```python
from build123d import *

# Parameters (mm, degrees)
F0_W     = 400
F0_H     = 80
F1_DEPTH = 7.5
F2_R     = 8
F3_W     = 12
F3_H     = 15
F3_W_2   = 15
F3_H_2   = 12
F4_DEPTH = 11.5
F5_R     = 5.5
F6_DEPTH = 25


# Not quite as in the source:
# - a pattern or mirror of a feature is missing from the dataset's text; its kind, count and spacing are read off the source's solid


with BuildPart() as f1:
    # F0 (on Top) → F1 (new body, symmetric)
    with BuildSketch(Plane.XY):
        Rectangle(F0_W, F0_H)
    extrude(amount=F1_DEPTH, both=True)

    # F2
    f2_edges = [f1.edges().sort_by_distance(p)[0] for p in [
        (-200, -40, 0),
        (200, -40, 0),
        (200, 40, 0),
        (-200, 40, 0),
    ]]
    fillet(f2_edges, radius=F2_R)

    # F3 (on Top) → F4 (join, symmetric)
    with BuildSketch(Plane.XY):
        with Locations((-186, -38.5)):
            Rectangle(F3_W, F3_H)
        with Locations((-186, 38.5)):
            Rectangle(F3_W, F3_H)
        with Locations((198.5, 0)):
            Rectangle(F3_W_2, F3_H_2)
    extrude(amount=F4_DEPTH, both=True)

    # F5 (on face) → F6 (cut)
    with BuildSketch(Plane.XY.offset(7.5)):
        Circle(F5_R)
    extrude(amount=-F6_DEPTH, mode=Mode.SUBTRACT)

    # F10 (on plane+point) → F11 (revolve)
    with BuildSketch(Plane.XZ.offset(-11)):
        with BuildLine():
            Line((-160, 40), (-160, 0))
            ThreePointArc((-160, 0), (-140, 20), (-160, 40))
        make_face()
    f11 = revolve(axis=Axis((-160, 11, 20), (0, 0, 1)))

    # F11_copies: F11 across plane
    add(f11.mirror(Plane(origin=(0, 0, 0), x_dir=(0, 0, 1), z_dir=(1, 0, 0))))


solid = f1.part
```
The model under review builds one solid part; all positions refer to its coordinate system, in mm. A direction names the side the tool comes from. Coordinates: 2 decimals unless noted, no trailing zeros. Order: outer loops, then holes, each group sorted by start corner. A loop starts at its lowest first (then second) coordinate and runs counter-clockwise, first axis right, second up. Notation, with made-up numbers: (23.25, -28) -> (82.25, -28) arc R22 cw to (82.25, -21) -> close; hole circle Ø4 at (14, 16). An arc over 180 degrees is marked (long way). Answer in a Markdown table with one row per item. Add a question column.
Item 1: Machinability: for faces 1 (the flat face through (-192, -40.3, -0.2)), 2 (the flat face through (200, 19, 0)), 3 (the flat face through (-192, 42, 0)), 4 (the flat face through (198, 0, 11.5)), which of the approach directions +Z, -Z, +X, -X, +Y, -Y give a long, thin tool a straight path to every point of the face, cutting with its end or side? Answer none if there is none.
Item 2: We need section D-D on y = 24.5. Write out the cut boundary in (x, z), plus the area to 3 significant figures.
Item 3: We need section A-A on x = 0. Write out the cut boundary in (y, z), plus the area to 4 significant figures.
Item 4: Clearance check with flat-ended pins moving along their axes: pin 1 (9.5 mm diameter, centred on x = -184.5, y = 41, fed in from +Z); pin 2 (3 mm diameter, centred on y = -1.5, z = 9.5, fed in from -X); pin 3 (6 mm diameter, centred on x = -47, y = -9.5, fed in from +Z). State where each tip first meets the part, or that it passes through.
Item 5: We need section C-C on z = 1. Write out the cut boundary in (x, y).
Item 6: To check wall thickness, follow probe 1 along Y at (x, z) = (0, 0); probe 2 along X at (y, z) = (2, 23); probe 3 along Z at (x, y) = (-79, -33.5). State the ranges of each line that lie inside material, in increasing order.
Item 7: We need section B-B on y = 0. Write out the cut boundary in (x, z), plus the area to 3 significant figures.
Final values:
| question | item | result |
|---|---|---|
| 1 | face 1 | -X, -Y |
| 1 | face 2 | +Z, -Z, +X, +Y |
| 1 | face 3 | -X, +Y |
| 1 | face 4 | +Z, +X, +Y, -Y |
| 2 | outline | (-200, -7.5) -> (200, -7.5) -> (200, 7.5) -> (167.84, 7.5) arc R14.76 ccw (long way) to (152.16, 7.5) -> (-152.16, 7.5) arc R14.76 ccw (long way) to (-167.84, 7.5) -> (-200, 7.5) -> close |
| 2 | area | 7,320 mm2 |
| 3 | outline | (-40, -7.5) -> (-5.5, -7.5) -> (-5.5, 7.5) -> (-40, 7.5) -> close; (5.5, -7.5) -> (40, -7.5) -> (40, 7.5) -> (5.5, 7.5) -> close |
| 3 | area | 1,035 mm2 |
| 4 | pin 1 | stops at z = 11.5 |
| 4 | pin 2 | stops at x = -173.42 |
| 4 | pin 3 | stops at z = 7.5 |
| 5 | outline | (-200, -32) arc R8 ccw to (-192, -40) -> (-192, -46) -> (-180, -46) -> (-180, -40) -> (192, -40) arc R8 ccw to (200, -32) -> (200, -6) -> (206, -6) -> (206, 6) -> (200, 6) -> (200, 32) arc R8 ccw to (192, 40) -> (-180, 40) -> (-180, 46) -> (-192, 46) -> (-192, 40) arc R8 ccw to (-200, 32) -> close; hole circle Ø11 at (0, 0) |
| 6 | probe 1 | y = -40 to -5.5, 5.5 to 40 |
| 6 | probe 2 | x = -177.61 to -142.39, 142.39 to 177.61 |
| 6 | probe 3 | z = -7.5 to 7.5 |
| 7 | outline | (-200, -7.5) -> (-5.5, -7.5) -> (-5.5, 7.5) -> (-148.92, 7.5) arc R16.7 ccw (long way) to (-171.08, 7.5) -> (-200, 7.5) -> close; (5.5, -7.5) -> (191, -7.5) -> (191, -11.5) -> (206, -11.5) -> (206, 11.5) -> (191, 11.5) -> (191, 7.5) -> (171.08, 7.5) arc R16.7 ccw (long way) to (148.92, 7.5) -> (5.5, 7.5) -> close |
| 7 | area | 7,670 mm2 |
